Autodesk Inventor part; units mm, degrees
ref_plane "Plano de trabajo1" through (0, 4.5, 0) normal (0, 1, 0) x (1, 0, 0)
ref_plane "YZ Plane" through (0, 0, 0) normal (1, 0, 0) x (0, 1, 0)
ref_plane "XZ Plane" through (0, 0, 0) normal (0, 1, 0) x (-1, 0, 0)
sketch "Boceto1" plane through (0, 0, 0) normal (0, 1, 0) x (-1, 0, 0)
  circle A0 centre (0, 0) radius 4
  circle A1 centre (0, 0) radius 1
  dimension "d0" = 8
  dimension "d7" = 2
extrude "Extrusión1" add sketch "Boceto1" along normal mid plane 12 contours A0 | A1
ref_plane "Plano de trabajo1" through (0, 4.5, 0) normal (0, 1, 0) x (1, 0, 0)
sketch "Boceto2" plane through (0, 4.5, 0) normal (0, 1, 0) x (1, 0, 0)
  circle A0 centre (0, 0) radius 4
  circle A1 centre (0, 0) radius 2.7
  dimension "d4" = 5.4
extrude "Extrusión2" cut sketch "Boceto2" against normal blind 1.5
mirror "Simetría1" about plane through (0, 0, 0) normal (0, 1, 0) of "Extrusión2"
shell "Vaciado2" thickness 0.6 removed faces 0
sketch "Boceto4" plane through (0, 6, 0) normal (0, 1, 0) x (1, 0, 0)
  circle A0 centre (0, 0) radius 1
  dimension "d14" = 2
extrude "Extrusión4" cut sketch "Boceto4" against normal through all
properties part number "antivibracion_3DPrint"
Design review of the part built by this model. Coordinates are the model's own, in mm. A direction names the side the tool comes from. Coordinates: 2 decimals unless noted, no trailing zeros. Loops run counter-clockwise (first coordinate to the right, second up) from the corner with the lowest first, then second, coordinate; pieces in that order, holes last. Notation, with made-up numbers: M 49.25,6.5 L 88.25,6.5 A21 cw 88.25,26.5 Z; hole C 32,74.5 d11. An arc over 180 degrees is marked long. One line per question, with ' | ' between items.
(1) We need section A-A (y = 0.75). Give the boundary of the cut face in (x, z).
Filled in:
outline: C 0,0 d8; hole C 0,0 d6.8
(2) We need section B-B (z = -2.25). Count the separate pieces of the cut face and the enclosed holes in it, and give its area (3 significant figures).
Filled in:
separate pieces: 1 | enclosed holes: 3 | area: 41.0 mm^2
(3) Machinability: for faces 5 (the face through (0.74, -5.25, -3.32)), 6 (the face through (0.867, -5.24, -3.905)), which of the approach directions +Z, -Z, +X, -X, +Y, -Y give a long, thin tool a straight path to every point of the face, cutting with its end or side? Answer none if there is none.
Filled in:
face 5: none | face 6: +Y, -Y
(4) We need section D-D (y = -4.25). Give the boundary of the cut face in (x, z).
Filled in:
outline: C 0,0 d5.4; hole C 0,0 d4.2
(5) Wall thickness on probe 1 along Y at (x, z) = (-2, -2.25); probe 2 along Y at (x, z) = (-1.25, 3.5); probe 3 along Y at (x, z) = (-1, -0.5): over which ranges is each line inside the solid? List them lowest first.
Filled in:
probe 1: y = -6 to -5.4, -5.1 to -4.5, -3 to -2.4, 2.4 to 3, 4.5 to 5.1, 5.4 to 6 | probe 2: y = -6 to -4.5, -3 to 3, 4.5 to 6 | probe 3: y = -6 to -5.4, 5.4 to 6
(6) Draft analysis for pull direction X (two halves, no side actions). For faces 1 (the face through (-0.217, -5.696, 0.976)), 2 (the face through (0.74, 5.25, -3.32)), 3 (the face through (-1, 6, -1)), 4 (the face through (-0.585, 3.76, 2.636)), state which applies: released by +X, released by -X, zero draft, split by the parting line, or undercut.
Filled in:
face 1: undercut | face 2: undercut | face 3: zero draft | face 4: split by the parting line
(7) For pin 1 Ø1.8 at (x, z) = (0, 0) entering from +Y; pin 2 Ø1.5 at (y, z) = (-1, -2.5) entering from +X; pin 3 Ø1 at (x, y) = (2, -2) entering from -Z, all flat-tipped, find the tip position at first contact; note any pin that passes through.
Filled in:
pin 1: passes through | pin 2: stops at x = 3.6 | pin 3: stops at z = -3.71
